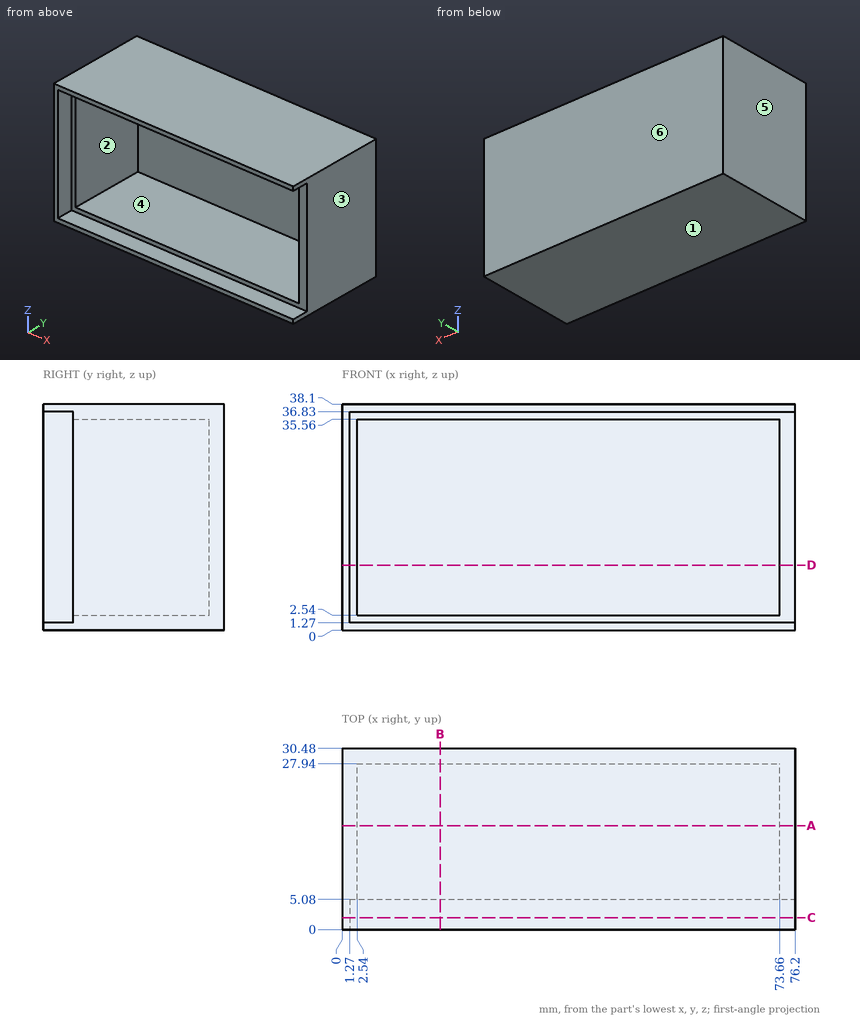
Could you check a few things on this drawing? It's one solid part, dimensions in mm from its lowest x, y, z. A direction names the side the tool comes from. Coordinates: 2 decimals unless noted, no trailing zeros. Order: outer loops, then holes, each group sorted by start corner. A loop starts at its lowest first (then second) coordinate and runs counter-clockwise, first axis right, second up. Notation, with made-up numbers: M 36.5,-4 L 73.5,-4 A25 cw 73.5,8 Z; hole C 79,4 d5. An arc over 180 degrees is marked long. Use one line per item in the form item = value. Start each with the question number.
1. We'd pull the mould along X, two halves only. Please class the marked faces 3, 4, 5 and 6: +X half, -X half, draft (parallel to the pull), parting line (faces both ways), or undercut.
2. On a 3-axis mill with a long thin cutter (end or side, diameter ignored), from which of +Z, -Z, +X, -X, +Y, -Y can I reach the whole of each face in a straight line? I mean the marked faces 1 and 2. Say none if no direction works.
3. Suppose I cut it at C-C on y = 2. Write out the boundary of the cut face in (x, z), then the cut area to 3 significant figures.
4. Suppose I cut it at A-A on y = 17.5. Write out the boundary of the cut face in (x, z).
5. Suppose I cut it at D-D on z = 11. Write out the boundary of the cut face in (x, y).
6. Please list where these lines run through material, in increasing order: line 1 (X direction, y = 9.5, z = 8); line 2 (Z direction, x = 66.5, y = 23); line 3 (Y direction, x = 64.5, z = 2).
7. For pin 1 (10.5 mm diameter, centred on x = 31, z = 17.5, fed in from -Y); pin 2 (6 mm diameter, centred on x = 21.5, z = 33.5, fed in from -Y); pin 3 (4 mm diameter, centred on y = 3, z = 25, fed in from +X), each with a flat end and sliding along its axis, tell me the tip position at first contact or that it passes through.
8. Suppose I cut it at B-B on x = 16.5. Write out the boundary of the cut face in (y, z).
Geometry says:
q1.face_3 = +X half
q1.face_4 = undercut
q1.face_5 = -X half
q1.face_6 = draft
q2.face_1 = -Z, +X, -X, +Y, -Y
q2.face_2 = -Y
q3.outline = M 0,0 L 76.2,0 L 76.2,1.27 L 1.27,1.27 L 1.27,36.83 L 76.2,36.83 L 76.2,38.1 L 0,38.1 Z
q3.area = 239 mm^2
q4.outline = M 0,0 L 76.2,0 L 76.2,38.1 L 0,38.1 Z; hole M 2.54,2.54 L 73.66,2.54 L 73.66,35.56 L 2.54,35.56 Z
q5.outline = M 0,0 L 1.27,0 L 1.27,5.08 L 2.54,5.08 L 2.54,27.94 L 73.66,27.94 L 73.66,5.08 L 76.2,5.08 L 76.2,30.48 L 0,30.48 Z
q6.line_1 = 0 to 2.54, 73.66 to 76.2
q6.line_2 = 0 to 2.54, 35.56 to 38.1
q6.line_3 = 5.08 to 30.48
q7.pin_1 = 27.94
q7.pin_2 = 5.08
q7.pin_3 = 1.27
q8.outline = M 0,0 L 30.48,0 L 30.48,38.1 L 0,38.1 L 0,36.83 L 5.08,36.83 L 5.08,35.56 L 27.94,35.56 L 27.94,2.54 L 5.08,2.54 L 5.08,1.27 L 0,1.27 Z
